The listing builds one solid part. Answer for the finished solid, in the listing's coordinates (mm). Face numbers are marked on the shaded views. A direction names the side the tool comes from. Round coordinates to 2 decimals unless told otherwise and drop trailing zeros. Write each loop counter-clockwise with the first axis right and the second up, starting at its lowest first coordinate (ties: lowest second). Pieces come first, ordered by that corner, then holes. Notation, with made-up numbers: (-3, 52) - (28, 52) arc R14 cw to (28, 78) - close; hole circle Ø6 at (69.5, 47.5). An arc over 180 degrees is marked (long way). Return JSON: item names as keys, results as strings. Group by question number.
(1) Which of the six approach directions +Z, -Z, +X, -X, +Y, -Y give full straight-line access (tool end or side, diameter ignored) to the marked faces 1 and 2?
(2) Section C-C, the plane z = -8.5 is taken. Write down the section's boundary in (x, y).
(3) Find the intervals of material crossed by line 1 along X through (y, z) = (19, 0); line 2 along Y through (x, z) = (7, -2.75); line 3 along X through (y, z) = (14, -1.5), in increasing order. Write a range as [from, to].
(4) Each of these flat-tipped pins is pushed along its axis until it touches: pin 1 (1.5 mm diameter, centred on x = 1.5, z = 0, fed in from -Y); pin 2 (2 mm diameter, centred on x = -2, y = 20, fed in from -Z). Where does it stop, or does it pass through?
(5) Determine the mould class of the marked faces 3, 4, 5 and 6 for opening direction X: +X half, -X half, draft (parallel to the pull), parting line (faces both ways), or undercut.
(6) Section A-A, the plane y = 12.75 is taken. Write down the section's boundary in (x, z).
(7) Section D-D, the plane y = 8 is taken. Write down the section's boundary in (x, z).
(8) Section B-B, the plane y = 4.5 is taken. Write down the section's boundary in (x, z).
Autodesk Inventor part; units mm, degrees
ref_plane "YZ Plane" through (0, 0, 0) normal (1, 0, 0) x (0, 1, 0)
ref_plane "XZ Plane" through (0, 0, 0) normal (0, 1, 0) x (-1, 0, 0)
ref_plane "XY Plane" through (0, 0, 0) normal (0, 0, 1) x (1, 0, 0)
sketch "Skizze6" plane through (0, 0, 0) normal (0, 0, 1) x (1, 0, 0)
  line L0 (0, 0) -> (6, 0)
  line L1 (6, 0) -> (6, 10)
  line L2 (6, 10) -> (10, 10)
  line L3 (10, 10) -> (10, 30)
  line L4 (10, 30) -> (0, 30)
  line L5 (0, 30) -> (0, 0)
  line L6 (0, 30) -> (0, 0)
  dimension "d34" = 20
  dimension "d35" = 12
  dimension "d36" = 20
  dimension "d37" = 30
revolve "Umdrehung1" add sketch "Skizze6" angle 360 about axis through (0, 30, 0) along (0, -1, 0)
sketch "Skizze7" plane through (0, 30, 0) normal (0, 1, 0) x (1, 0, 0)
  circle A0 centre (0, 0) radius 10
hole "Bohrung5" at (0, 30, 0) direction (0, -1, 0) diameter 6 end through all
sketch "Skizze8" plane through (0, 30, 0) normal (0, 1, 0) x (1, 0, 0)
  line L0 (-8.5, -5.2678) -> (-8.5, 5.2678)
  circle A0 centre (0, 0) radius 10
  line L1 (0, 10) -> (0, -10)
  arc A1 (-8.5, 5.2678) -> (-8.5, -5.2678) centre (0, 0) ccw
  line L2 (8.5, -5.2678) -> (8.5, 5.2678)
  arc A2 (8.5, -5.2678) -> (8.5, 5.2678) centre (0, 0) ccw
  dimension "d46" = 17
extrude "Extrusion2" cut sketch "Skizze8" against normal up to surface (20 mm away) contours A0 L0 | L2 A0
chamfer "Fase1" distance 0.5 angle 45 1 edges at (-6, 0, 0)
sketch "Skizze9" plane through (0, 0, 0) normal (1, 0, 0) x (0, 1, 0)
  line L0 (10, 6) -> (0.5, 6)
  line L1 (10, -5.2678) -> (10, 5.2678)
  line L2 (10, 6) -> (10, 4.75)
  line L3 (10, 5.2678) -> (10, -5.2678)
  line L4 (10, 4.75) -> (9, 4.75)
  line L5 (9, 4.75) -> (6.8349, 6)
  line L6 (6.8349, 6) -> (10, 6)
  line L7 (0, 0) -> (30, 0)
  line L8 (30, 3) -> (30, -3)
  dimension "d52" = 9.5
  dimension "d53" = 30
  dimension "d54" = 1
revolve "Umdrehung2" cut sketch "Skizze9" angle 360 about axis through (0, 0, 0) along (0, 1, 0)
fillet "Rundung1" radius 0.3 2 edges at (0, 10, -4.75) (0, 9, -4.75)
thread "Gewinde1"
properties part number "106.015.01_Justage_Vereinzelung" material "Aluminium 6061"
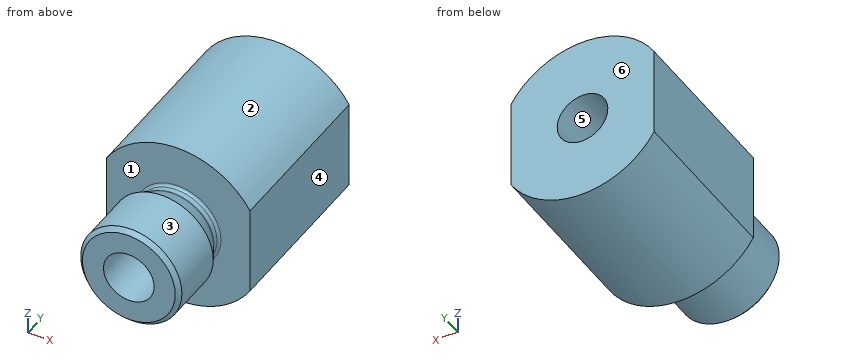
Working result:
{
 "1": {"face 1": "none", "face 2": "+Z, +Y, -Y"},
 "2": {"outline": "(-5.27, 10) - (5.27, 10) - (5.27, 30) - (-5.27, 30) - close"},
 "3": {"line 1": "x = [-8.5, -3], [3, 8.5]", "line 2": "y = [10, 30]", "line 3": "x = [-8.5, -2.6], [2.6, 8.5]"},
 "4": {"pin 1": "passes through", "pin 2": "stops at z = -9.95"},
 "5": {"face 3": "parting line", "face 4": "+X half", "face 5": "undercut", "face 6": "draft"},
 "6": {"outline": "(-8.5, -5.27) arc R10 ccw to (8.5, -5.27) - (8.5, 5.27) arc R10 ccw to (-8.5, 5.27) - close; hole circle Ø6 at (0, 0)"},
 "7": {"outline": "circle Ø10.65 at (0, 0); hole circle Ø6 at (0, 0)"},
 "8": {"outline": "circle Ø12 at (0, 0); hole circle Ø6 at (0, 0)"}
}
